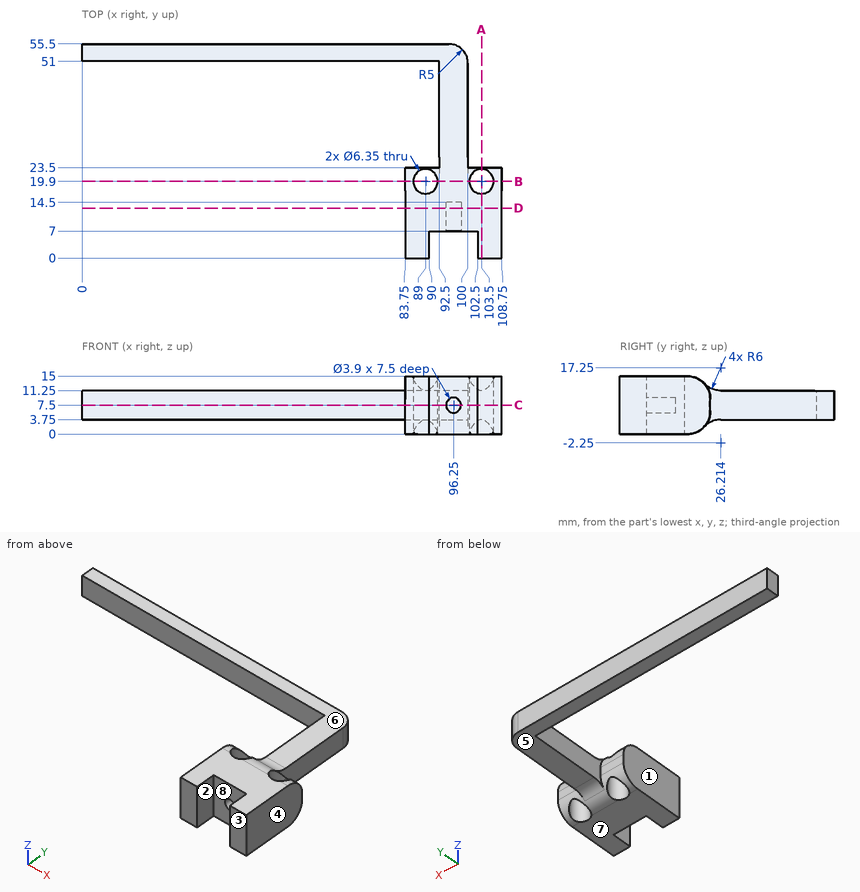
Check sheet for the drawn part. Datum: minimum x, y, z corner. Units: mm. A direction names the side the tool comes from. Coordinates: 2 decimals unless noted, no trailing zeros. Loops run counter-clockwise (first coordinate to the right, second up) from the corner with the lowest first, then second, coordinate; pieces in that order, holes last. Notation, with made-up numbers: (-25.5, -2.75) -> (-19.5, -2.75) arc R21 cw to (-19.5, 17.25) -> close; hole circle Ø4 at (-31.75, 23.5). An arc over 180 degrees is marked (long way). Answer in a Markdown table with one row per item.
1) Scan lines: line 1 along X through (y, z) = (19.9, 5) (3 decimals); line 2 along X through (y, z) = (10.5, 7.5); line 3 along X through (y, z) = (5.5, 10.5). Record each from-to range of solid material in increasing order. Write a range as from..to.
The answers:
| item | result |
|---|---|
| line 1 | x = 83.75..85.825, 92.175..100.325, 106.675..108.75 |
| line 2 | x = 83.75..94.3, 98.2..108.75 |
| line 3 | x = 83.75..90, 102.5..108.75 |
2) Section check B-B (y = 19.9). Give the number of separate pieces and of enclosed holes in the cut face, and give its area (3 significant figures).
The answers:
| item | result |
|---|---|
| separate pieces | 3 |
| enclosed holes | 0 |
| area | 172 mm2 |
3) Access from +Z, -Z, +X, -X, +Y, -Y to the whole of each face (thin tool, end or side, straight path). Record for the marked faces 5, 6, 7 and 8.
The answers:
| item | result |
|---|---|
| face 5 | -Z, +X, -X, +Y |
| face 6 | +Z, +X, -X, +Y |
| face 7 | -Z, +X, -X, +Y, -Y |
| face 8 | +Z, -Z, -Y |
4) Section check A-A (x = 103.5). Record the cut outline in (y, z) (3 decimals).
The answers:
| item | result |
|---|---|
| outline | (0, 0) -> (16.725, 0) -> (16.725, 15) -> (0, 15) -> close; (23.075, 3.782) arc R6 ccw to (23.5, 6) -> (23.5, 9) arc R6 ccw to (23.075, 11.218) -> close |
5) Section check C-C (z = 7.5). Record the cut outline in (x, y) (3 decimals).
The answers:
| item | result |
|---|---|
| outline | (0, 51) -> (92.5, 51) -> (92.5, 23.5) -> (83.75, 23.5) -> (83.75, 0) -> (90, 0) -> (90, 7) -> (94.3, 7) -> (94.3, 14.5) -> (98.2, 14.5) -> (98.2, 7) -> (102.5, 7) -> (102.5, 0) -> (108.75, 0) -> (108.75, 23.5) -> (100, 23.5) -> (100, 50.5) arc R5 ccw to (95, 55.5) -> (0, 55.5) -> close; hole circle Ø6.35 at (89, 19.9); hole circle Ø6.35 at (103.5, 19.9) |
6) Draft check along X on the marked faces 1, 2, 3 and 4. Enter one of: released by +X, released by -X, zero draft, split by the parting line, or undercut.
The answers:
| item | result |
|---|---|
| face 1 | released by -X |
| face 2 | undercut |
| face 3 | zero draft |
| face 4 | released by +X |
7) Depth check by flat-ended pin: P1, Ø7.5, axis at y = 10, z = 10, coming from the -X side; P2, Ø8, axis at x = 59.5, z = 8.5, coming from the -Y side; P3, Ø7.5, axis at x = 103.5, y = 19.9, coming from the -Z side; P4, Ø5.5, axis at y = 39, z = 8, coming from the -X side. Enter the tip coordinate at first touch or a pass-through.
The answers:
| item | result |
|---|---|
| P1 | stops at x = 83.75 |
| P2 | stops at y = 51 |
| P3 | stops at z = 0 |
| P4 | stops at x = 92.5 |
8) Section check D-D (y = 13). Record the cut outline in (x, z), and give its area (3 significant figures).
The answers:
| item | result |
|---|---|
| outline | (83.75, 0) -> (108.75, 0) -> (108.75, 15) -> (83.75, 15) -> close; hole circle Ø3.9 at (96.25, 7.5) |
| area | 363 mm2 |
